Geometry check sheet. Reference: the model listing, model coordinates, mm. Face numbers are marked on the shaded views. A direction names the side the tool comes from. Round coordinates to 2 decimals unless told otherwise and drop trailing zeros. Order: outer loops, then holes, each group sorted by start corner. A loop starts at its lowest first (then second) coordinate and runs counter-clockwise, first axis right, second up.
(1) Cross-section at B-B on x = -42. Enter the section's corners in (y, z), and give its area (3 significant figures).
(2) Thickness scan on L1, parallel to Z at x = -81.5, y = 9.25; L2, parallel to Y at x = -37.5, z = 20; L3, parallel to X at y = 8.75, z = 18.75. Record the ranges inside material, lowest first.
(3) Cross-section at C-C on z = 4.75. Enter the section's corners in (x, y), and give its area (3 significant figures).
(4) Gauge pin test, flat ends, axial feed: P1, Ø9, axis at x = -52.5, y = 12, coming from the +Z side; P2, Ø4, axis at x = -54.5, z = 15, coming from the +Y side; P3, Ø8, axis at y = 11, z = 21.5, coming from the +X side. Record the tip position at first contact, or that the pin passes through.
(5) Set-up check for the marked faces 1 and 2: record each of +Z, -Z, +X, -X, +Y, -Y from which the full face is reachable in a straight line by a thin tool's end or side.
(6) Cross-section at A-A on y = 13. Enter the section's corners in (x, z), and give its area (3 significant figures).
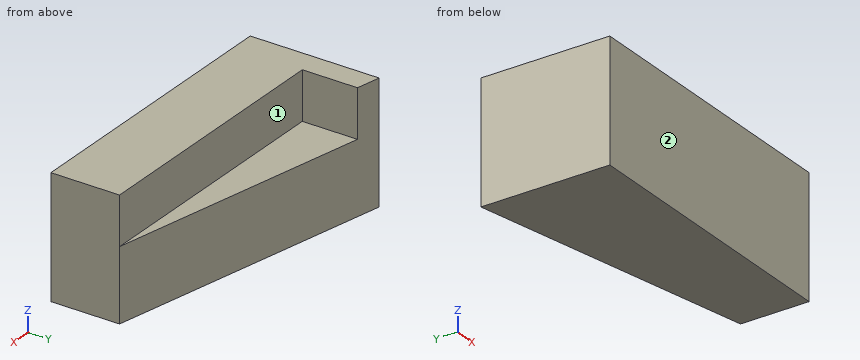
from build123d import *

# Parameters (mm, degrees)
F1_DEPTH = 15
F3_DEPTH = 10
F4_DEPTH = 3
F5_DEPTH = 5


with BuildPart() as f1:
    # F0 (on Top) → F1 (new body)
    with BuildSketch(Plane.XY):
        Polygon((30, 6.25), (30, 0), (60, 0), (60, 12.5), align=None)
        Polygon((60, 12.5), (60, 0), (90, 0), (90, 18.75), align=None)
    extrude(amount=F1_DEPTH)

    # F2 (on face) → F3 (join)
    with BuildSketch(Plane.XY.offset(15)):
        Polygon((30, 0), (90, 0), (90, 18.75), (85.0000008941, 17.7083335196), (85.0000008941, 6.25), (30, 6.25), align=None)
    extrude(amount=F3_DEPTH)

    # F4 (add): a face of the model
    f4_faces = [f1.faces().sort_by_distance(p)[0] for p in [
        (60, 0, 12.5),
    ]]
    extrude(f4_faces, amount=F4_DEPTH)

    # F5 (add): a face of the model
    f5_faces = [f1.faces().sort_by_distance(p)[0] for p in [
        (60, -3, 12.5),
    ]]
    extrude(f5_faces, amount=F5_DEPTH)


with BuildPart() as f6_1:
    # F6: instance of F1
    add(f1.part.mirror(Plane.YZ))


solid = f6_1.part
Found:
1. outline: (-8, 0) - (8.75, 0) - (8.75, 15) - (6.25, 15) - (6.25, 25) - (-8, 25) - close
1. area: 394 mm2
2. L1: z = 0 to 15
2. L2: y = -8 to 6.25
2. L3: x = -90 to -85
3. outline: (-90, -8) - (-30, -8) - (-30, 6.25) - (-90, 18.75) - close
3. area: 1,230 mm2
4. P1: stops at z = 15
4. P2: stops at y = 11.77
4. P3: stops at x = -85
5. face 1: +Z, +X, +Y
5. face 2: +Z, -Z, +X, -X, -Y
6. outline: (-90, 0) - (-62.4, 0) - (-62.4, 15) - (-85, 15) - (-85, 25) - (-90, 25) - close
6. area: 464 mm2
